Input: part model. Units: mm. Frame: model coordinates. Face numbers are marked on the shaded views. A direction names the side the tool comes from. Round coordinates to 2 decimals unless told otherwise and drop trailing zeros. Loops run counter-clockwise (first coordinate to the right, second up) from the corner with the lowest first, then second, coordinate; pieces in that order, holes last. Notation, with made-up numbers: (12, -7) - (69, -7) arc R16 cw to (69, 21) - close; hole circle Ø3 at (-29, 40). An arc over 180 degrees is marked (long way). One line per question, with ' | ' between items. Start each with the question number.
Item 1: Section D-D, the plane x = 7.25. Return loops of the section in (y, z), plus the area to 3 significant figures.
Item 2: Section A-A, the plane z = 6. Return loops of the section in (x, y), plus the area to 3 significant figures.
Item 3: Draft query along X for the marked faces 3, 4 and 5. Return one class per face: pulls with the +X half, pulls with the -X half, needs draft (parallel to the pull), parting line crosses it, or undercut.
Item 4: Set-up query: the marked faces 1 and 2. Return all of +Z, -Z, +X, -X, +Y, -Y with unobstructed straight access to the full face (end or side cutting, diameter ignored); none if empty.
Item 5: Material intervals for line 1 along Y through (x, z) = (0, 3.25); line 2 along Y through (x, z) = (0, 2.25); line 3 along Y through (x, z) = (5.5, 5.25), sorted ascending.
Item 6: Section C-C, the plane y = 3.75. Return loops of the section in (x, z), plus the area to 3 significant figures.
Item 7: First-contact query: pin 1 (4 mm diameter, centred on x = 7.5, z = 1, fed in from +Y) (3 decimals); pin 2 (1.5 mm diameter, centred on x = -0.5, z = 1.5, fed in from -Y); pin 3 (0.6 mm diameter, centred on y = 1, z = 1, fed in from +X). Flat tips, straight axial feed; report the tip coordinate or a pass-through.
Item 8: Section B-B, the plane x = 0. Return loops of the section in (y, z).
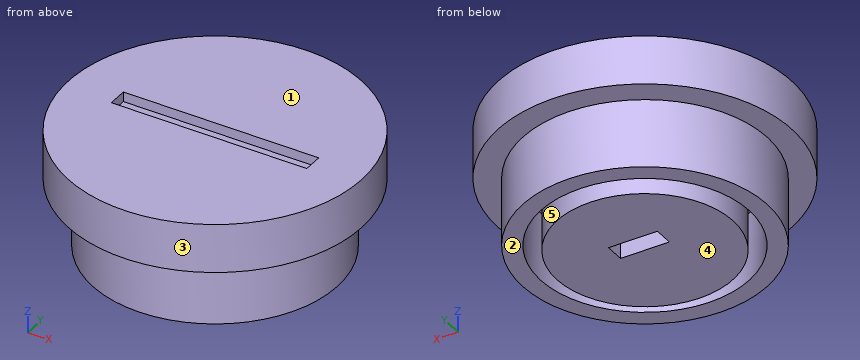
```python
from build123d import *

# Parameters (mm, degrees)
SKETCH_1_R          = 12.5
SKETCH_1_R_2        = 10.65
EXTRUDE_1_DEPTH     = 7
SKETCH_2_R          = 15
EXTRUDE_2_DEPTH     = 5
SKETCH_4_R          = 9
EXTRUDE_3_DEPTH     = 7.5
SKETCH_5_W          = 20
SKETCH_5_H          = 2
CUT_EXTRUDE_1_DEPTH = 1
SKETCH_6_W          = 5
SKETCH_6_H          = 2
CUT_EXTRUDE_2_DEPTH = 3


with BuildPart() as part:
    # 스케치1 → 보스-돌출1 (new body)
    with BuildSketch(Plane.XY):
        Circle(SKETCH_1_R)
        Circle(SKETCH_1_R_2, mode=Mode.SUBTRACT)
    extrude(amount=EXTRUDE_1_DEPTH)

    # 스케치2 → 보스-돌출2 (add)
    with BuildSketch(Plane.XY.offset(7)):
        Circle(SKETCH_2_R)
    extrude(amount=EXTRUDE_2_DEPTH)

    # 스케치4 → 보스-돌출3 (add)
    with BuildSketch(Plane(origin=(0, 0, 7), x_dir=(-1, 0, 0), z_dir=(0, 0, -1))):
        with Locations(Location((0, 0, 0), (0, 0, 180))):
            Circle(SKETCH_4_R)
    extrude(amount=EXTRUDE_3_DEPTH)

    # 스케치5 → 컷-돌출1 (cut)
    with BuildSketch(Plane.XY.offset(12)):
        Rectangle(SKETCH_5_W, SKETCH_5_H)
    extrude(amount=-CUT_EXTRUDE_1_DEPTH, mode=Mode.SUBTRACT)

    # 스케치6 → 컷-돌출2 (cut)
    with BuildSketch(Plane(origin=(0, 0, -0.5), x_dir=(-1, 0, 0), z_dir=(0, 0, -1))):
        with Locations((0, 1)):
            Rectangle(SKETCH_6_W, SKETCH_6_H)
    extrude(amount=-CUT_EXTRUDE_2_DEPTH, mode=Mode.SUBTRACT)


solid = part.part
```
Return value:
1) outline: (-13.13, 7) - (-10.18, 7) - (-10.18, 0) - (-7.8, 0) - (-7.8, 7) - (-5.33, 7) - (-5.33, -0.5) - (5.33, -0.5) - (5.33, 7) - (7.8, 7) - (7.8, 0) - (10.18, 0) - (10.18, 7) - (13.13, 7) - (13.13, 12) - (1, 12) - (1, 11) - (-1, 11) - (-1, 12) - (-13.13, 12) - close | area: 243 mm2
2) outline: circle Ø25 at (0, 0); circle Ø18 at (0, 0); hole circle Ø21.3 at (0, 0) | area: 389 mm2
3) face 3: parting line crosses it | face 4: needs draft | face 5: undercut
4) face 1: +Z, +X, -X, +Y, -Y | face 2: -Z
5) line 1: -12.5 to -10.65, -9 to 9, 10.65 to 12.5 | line 2: -12.5 to -10.65, -9 to 0, 2 to 9, 10.65 to 12.5 | line 3: -11.22 to -9.12, -7.12 to 7.12, 9.12 to 11.22
6) outline: (-14.52, 7) - (-11.92, 7) - (-11.92, 0) - (-9.97, 0) - (-9.97, 7) - (-8.18, 7) - (-8.18, -0.5) - (8.18, -0.5) - (8.18, 7) - (9.97, 7) - (9.97, 0) - (11.92, 0) - (11.92, 7) - (14.52, 7) - (14.52, 12) - (-14.52, 12) - close | area: 295 mm2
7) pin 1: y = 11.225 | pin 2: y = -12.5 | pin 3: x = 12.48
8) outline: (-15, 7) - (-12.5, 7) - (-12.5, 0) - (-10.65, 0) - (-10.65, 7) - (-9, 7) - (-9, -0.5) - (0, -0.5) - (0, 2.5) - (2, 2.5) - (2, -0.5) - (9, -0.5) - (9, 7) - (10.65, 7) - (10.65, 0) - (12.5, 0) - (12.5, 7) - (15, 7) - (15, 12) - (1, 12) - (1, 11) - (-1, 11) - (-1, 12) - (-15, 12) - close
